```python
from build123d import *

# Parameters (mm, degrees)
F1_DEPTH       = 120.65
F3_D           = 20.6375
F3_CBORE_D     = 30.1752
F3_CBORE_DEPTH = 28.448
F4_R           = 1.524


# Not quite as in the source:
# - a length typed as a fraction of an inch, garbled in the dataset ("3 / 203.2 mm" for 3/8 in), is restored


with BuildPart() as f1:
    # F0 (on Top) → F1 (new body, symmetric)
    with BuildSketch(Plane.XY):
        Polygon((95.25, 44.45), (-95.25, 44.45), (-95.25, 31.75), (-57.15, 31.75), (-57.15, -31.75), (-95.25, -31.75), (-95.25, -44.45), (95.25, -44.45), align=None)
    extrude(amount=F1_DEPTH, both=True)

    # F3 (through all)
    with Locations(Plane.YZ.offset(95.25)):
        with Locations((0, 63.5), (0, -63.5)):
            CounterBoreHole(F3_D / 2, F3_CBORE_D / 2, F3_CBORE_DEPTH)

    # F4
    f4_edges = [f1.edges().sort_by_distance(p)[0] for p in [
        (-57.15, -31.75, 0),
        (-57.15, 31.75, 0),
    ]]
    fillet(f4_edges, radius=F4_R)


solid = f1.part
```
Can you work these out from the model? Positions are in its coordinate system, mm. A direction names the side the tool comes from. Give positions to 0.01 mm unless a question says otherwise; leave off trailing zeros. Write each loop counter-clockwise with the first axis right and the second up, starting at its lowest first coordinate (ties: lowest second). Pieces come first, ordered by that corner, then holes. Notation, with made-up numbers: (58.25, -5) - (117.25, -5) arc R21 ccw to (117.25, 17) - close; hole circle Ø4 at (-31.75, -25.5). An arc over 180 degrees is marked (long way). Write item = value, one per line. Start each with the question number.
1. Imagine slicing it at A-A (z = -63.5). Please give me the cut outline in (x, y), and give its area (3 significant figures).
2. Imagine slicing it at D-D (z = -90.5). Please give me the cut outline in (x, y).
3. Imagine slicing it at C-C (y = 0). Please give me the cut outline in (x, z).
4. On a 3-axis mill with a long thin cutter (end or side, diameter ignored), from which of +Z, -Z, +X, -X, +Y, -Y can I reach the whole of each face in a straight line? I mean faces 5 (the face through (-1, -44.45, 2)), 6 (the face through (-57.15, 0, 2)), 7 (the face through (66.802, 10, 60)). Say none if no direction works.
5. Thinking about a two-plate mould opening in Z: for faces 1 (the face through (-77, -31.75, 2)), 2 (the face through (3.96, 1.34, 73.73)), 3 (the face through (20, 1, -120.65)), 4 (the face through (20, 1, 120.65)), which applies, released by +Z, released by -Z, zero draft, split by the parting line, or undercut?
6. Imagine slicing it at B-B (x = -62.5). Please give me the cut outline in (y, z), and give its area (3 significant figures).
7. Please list where these lines run through material, in increasing order: line 1 (Z direction, x = 72.5, y = 0); line 2 (Y direction, x = -77.5, z = 4); line 3 (Z direction, x = -16, y = -9.5).
8. For pin 1 (8 mm diameter, centred on y = 24.5, z = -2.5, fed in from -X), with a flat end and sliding along its axis, tell me the tip position at first contact or that it passes through.
Worked answers:
q1.outline = (-95.25, -44.45) - (95.25, -44.45) - (95.25, -15.09) - (66.8, -15.09) - (66.8, -10.32) - (-57.15, -10.32) - (-57.15, -30.23) arc R1.52 cw to (-58.67, -31.75) - (-95.25, -31.75) - close; (-95.25, 31.75) - (-58.67, 31.75) arc R1.52 cw to (-57.15, 30.23) - (-57.15, 10.32) - (66.8, 10.32) - (66.8, 15.09) - (95.25, 15.09) - (95.25, 44.45) - (-95.25, 44.45) - close
q1.area = 11,100 mm2
q2.outline = (-95.25, -44.45) - (95.25, -44.45) - (95.25, 44.45) - (-95.25, 44.45) - (-95.25, 31.75) - (-58.67, 31.75) arc R1.52 cw to (-57.15, 30.23) - (-57.15, -30.23) arc R1.52 cw to (-58.67, -31.75) - (-95.25, -31.75) - close
q3.outline = (-57.15, -120.65) - (95.25, -120.65) - (95.25, -78.59) - (66.8, -78.59) - (66.8, -73.82) - (-57.15, -73.82) - close; (-57.15, -53.18) - (66.8, -53.18) - (66.8, -48.41) - (95.25, -48.41) - (95.25, 48.41) - (66.8, 48.41) - (66.8, 53.18) - (-57.15, 53.18) - close; (-57.15, 73.82) - (66.8, 73.82) - (66.8, 78.59) - (95.25, 78.59) - (95.25, 120.65) - (-57.15, 120.65) - close
q4.face_5 = +Z, -Z, +X, -X, -Y
q4.face_6 = +Z, -Z, -X
q4.face_7 = +X
q5.face_1 = zero draft
q5.face_2 = undercut
q5.face_3 = released by -Z
q5.face_4 = released by +Z
q6.outline = (-44.45, -120.65) - (-31.75, -120.65) - (-31.75, 120.65) - (-44.45, 120.65) - close; (31.75, -120.65) - (44.45, -120.65) - (44.45, 120.65) - (31.75, 120.65) - close
q6.area = 6,130 mm2
q7.line_1 = -120.65 to -78.59, -48.41 to 48.41, 78.59 to 120.65
q7.line_2 = -44.45 to -31.75, 31.75 to 44.45
q7.line_3 = -120.65 to -67.53, -59.47 to 59.47, 67.53 to 120.65
q8.pin_1 = -57.15
